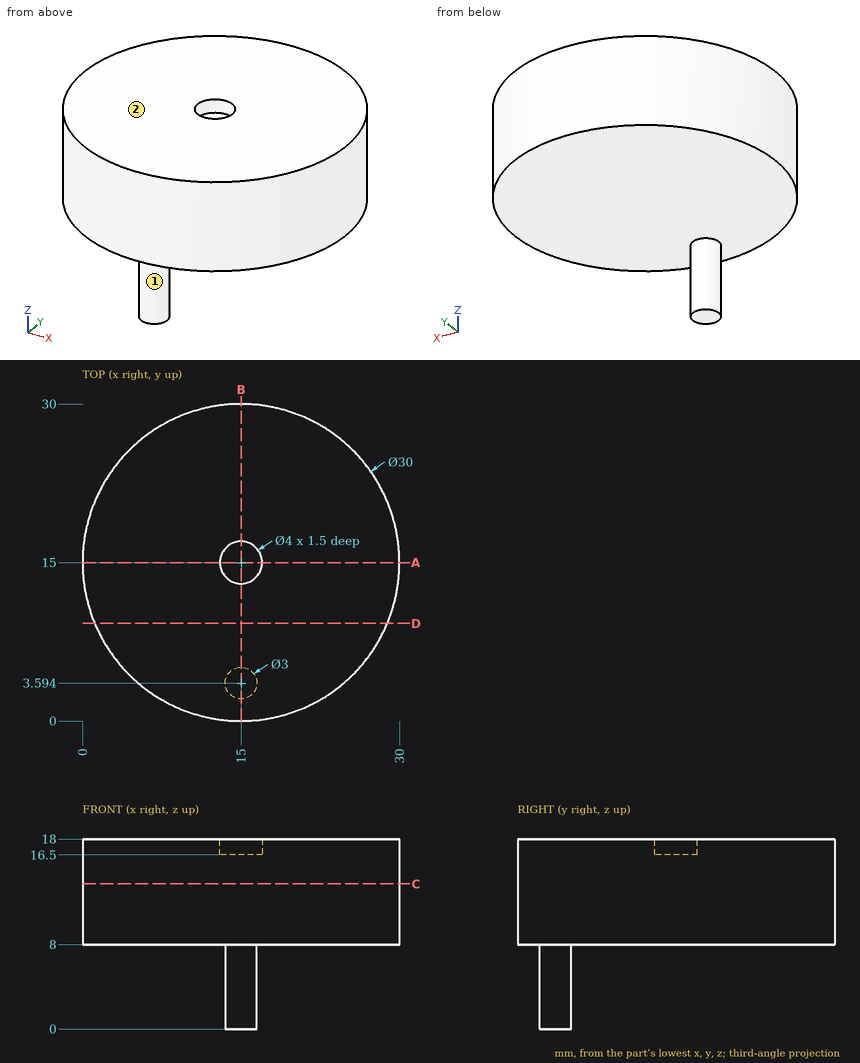
Geometry check sheet. Reference: drawing and pictorial views, mm from the part's lowest x, y, z. A direction names the side the tool comes from. Coordinates: 2 decimals unless noted, no trailing zeros. Order: outer loops, then holes, each group sorted by start corner. A loop starts at its lowest first (then second) coordinate and runs counter-clockwise, first axis right, second up.
Item 1: Material ranges on L1, parallel to Y at x = 15, z = 17.1; L2, parallel to Z at x = 7.25, y = 13; L3, parallel to Y at x = 18, z = 13.25, recorded low to high.
Filled in:
L1: y = 0 to 13, 17 to 30
L2: z = 8 to 18
L3: y = 0.3 to 29.7
Item 2: Section check B-B, the plane x = 15. Enter the section's corners in (y, z), then the cut area to 3 significant figures.
Filled in:
outline: (0, 8) - (2.09, 8) - (2.09, 0) - (5.09, 0) - (5.09, 8) - (30, 8) - (30, 18) - (17, 18) - (17, 16.5) - (13, 16.5) - (13, 18) - (0, 18) - close
area: 318 mm2
Item 3: Section check D-D, the plane y = 9.25. Enter the section's corners in (x, z).
Filled in:
outline: (1.15, 8) - (28.85, 8) - (28.85, 18) - (1.15, 18) - close
Item 4: Access from +Z, -Z, +X, -X, +Y, -Y to the whole of each face (thin tool, end or side, straight path). Record for the marked faces 1 and 2.
Filled in:
face 1: -Z
face 2: +Z, +X, -X, +Y, -Y
Item 5: Section check C-C, the plane z = 13.75. Enter the section's corners in (x, y), then the cut area to 3 significant figures.
Filled in:
outline: circle Ø30 at (15, 15)
area: 707 mm2
Item 6: Depth check by flat-ended pin: pin 1 (10 mm diameter, centred on x = 7, z = 14.5, fed in from -Y); pin 2 (4 mm diameter, centred on x = 3, z = 12.5, fed in from -Y); pin 3 (3 mm diameter, centred on x = 5.5, y = 11, fed in from -Z). Enter the tip coordinate at first touch or a pass-through.
Filled in:
pin 1: stops at y = 0.3
pin 2: stops at y = 3.82
pin 3: stops at z = 8
Item 7: Section check A-A, the plane y = 15. Enter the section's corners in (x, z), then the cut area to 3 significant figures.
Filled in:
outline: (0, 8) - (30, 8) - (30, 18) - (17, 18) - (17, 16.5) - (13, 16.5) - (13, 18) - (0, 18) - close
area: 294 mm2
